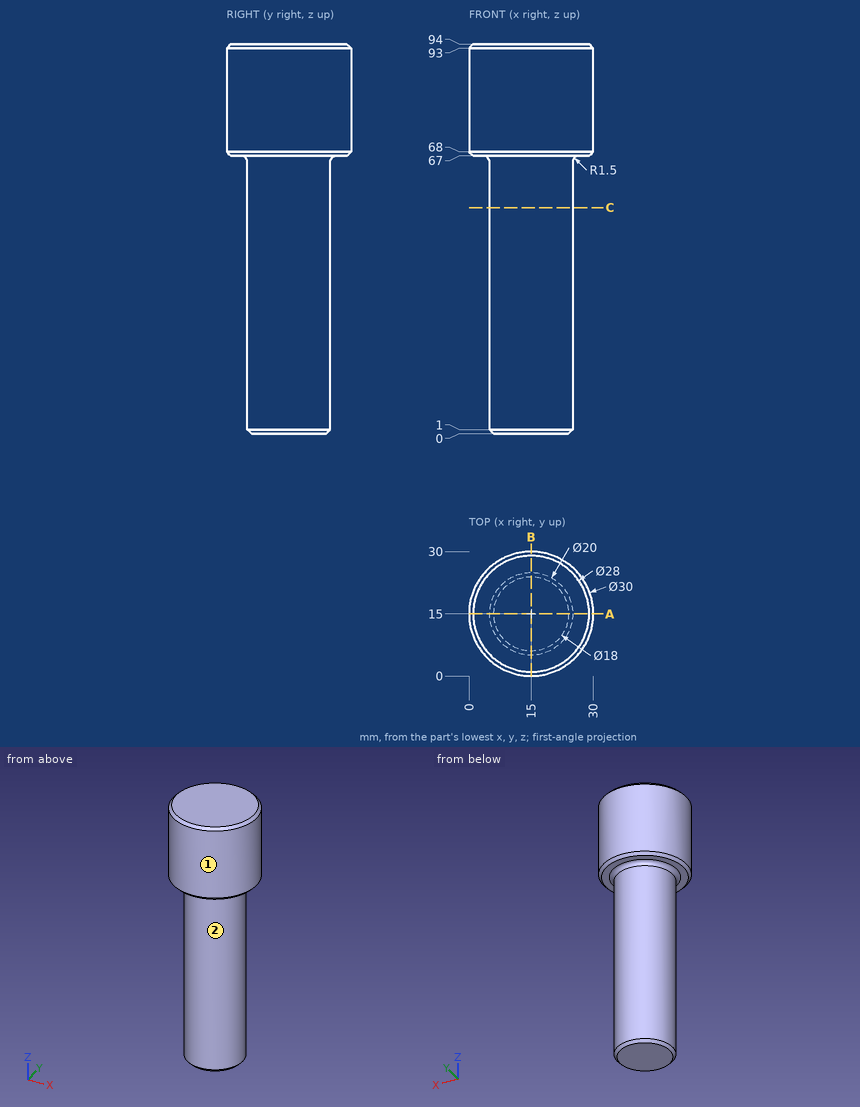
Source: three-view drawing plus pictorial views. Frame: mm from the lowest corner of the part. A direction names the side the tool comes from. Round coordinates to 2 decimals unless told otherwise and drop trailing zeros. Order: outer loops, then holes, each group sorted by start corner. A loop starts at its lowest first (then second) coordinate and runs counter-clockwise, first axis right, second up. Notation, with made-up numbers: (26, 61.5) -> (81, 61.5) arc R22 ccw to (81, 100.5) -> close; hole circle Ø11 at (-10.5, 17). An arc over 180 degrees is marked (long way). Use one line per item in the form item = value.
(1) Section C-C on z = 54.5. Return loops of the section in (x, y), and give its area (3 significant figures).
Results list:
outline = circle Ø20 at (15, 15)
area = 314 mm^2
(2) Section A-A on y = 15. Return loops of the section in (x, z).
Results list:
outline = (0, 68) -> (1, 67) -> (3.5, 67) arc R1.5 cw to (5, 65.5) -> (5, 1) -> (6, 0) -> (24, 0) -> (25, 1) -> (25, 65.5) arc R1.5 cw to (26.5, 67) -> (29, 67) -> (30, 68) -> (30, 93) -> (29, 94) -> (1, 94) -> (0, 93) -> close
(3) Ray query, probe 1 along Z at (x, y) = (6.25, 6.25); probe 2 along Y at (x, z) = (15, 52.5); probe 3 along Y at (x, z) = (17, 89). Return the intervals inside material, ascending. Write a range as [from, to].
Results list:
probe_1 = [67, 94]
probe_2 = [5, 25]
probe_3 = [0.13, 29.87]
(4) Access query for the marked faces 1 and 2. Directions: +Z, -Z, +X, -X, +Y, -Y. A direction counts if a zero-diameter tool reaches every point of the face in a straight line with its end or side. Return the directions, or none.
Results list:
face_1 = +Z, -Z
face_2 = -Z
(5) First-contact query: pin 1 Ø6 at (y, z) = (26, 46) entering from +X; pin 2 Ø1 at (y, z) = (21.5, 55) entering from -X; pin 3 Ø8 at (y, z) = (16, 66) entering from +X; pin 4 Ø1 at (y, z) = (15.5, 55.5) entering from -X. Flat tips, straight axial feed; report the tip coordinate or a pass-through.
Results list:
pin_1 = 21
pin_2 = 7
pin_3 = 30
pin_4 = 5
